Model file for the job. Use its own axes, mm. Face numbers are marked on the shaded views. A direction names the side the tool comes from. Coordinates: 2 decimals unless noted, no trailing zeros. Order: outer loops, then holes, each group sorted by start corner. A loop starts at its lowest first (then second) coordinate and runs counter-clockwise, first axis right, second up. Notation, with made-up numbers: M 84,5.25 L 128,5.25 A30 cw 128,38.25 Z; hole C 63,-14.75 d8. An arc over 180 degrees is marked long. Return JSON: item names as keys, results as strings.
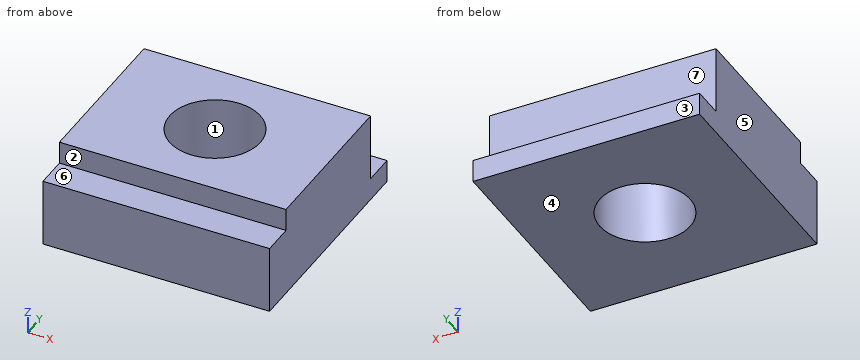
```python
from build123d import *

# Parameters (mm, degrees)
F0_W     = 50
F0_H     = 20
F1_DEPTH = 50
F2_W     = 7
F2_H     = 5
F2_H_2   = 15
F3_DEPTH = 50
F4_R     = 10
F5_DEPTH = 20


with BuildPart() as f1:
    # F0 (on Right) → F1 (new body)
    with BuildSketch(Plane.YZ):
        with Locations((25, 10)):
            Rectangle(F0_W, F0_H)
    extrude(amount=F1_DEPTH)

    # F2 (on face) → F3 (cut)
    with BuildSketch(Plane.YZ.offset(50)):
        with Locations((3.5, 17.5)):
            Rectangle(F2_W, F2_H)
        with Locations((46.5, 12.5)):
            Rectangle(F2_W, F2_H_2)
    extrude(amount=-F3_DEPTH, mode=Mode.SUBTRACT)

    # F4 (on face) → F5 (cut)
    with BuildSketch(Plane.XY.offset(20)):
        with Locations((25, 25)):
            Circle(F4_R)
    extrude(amount=-F5_DEPTH, mode=Mode.SUBTRACT)


solid = f1.part
```
Item 1: Drop flat-ended pins along their axis: pin 1 Ø16 at (x, y) = (25, 25) entering from +Z; pin 2 Ø2 at (x, z) = (27, 18) entering from -Y; pin 3 Ø5.5 at (x, y) = (34, 47.5) entering from +Z; pin 4 Ø2 at (x, y) = (34.5, 3) entering from +Z. Give the stop position or say it passes through.
Check result:
{"pin 1": "passes through", "pin 2": "stops at y = 7", "pin 3": "stops at z = 5", "pin 4": "stops at z = 15"}
Item 2: Saw through at A-A (y = 25). Write the cut outline in (x, z), and give its area (3 significant figures).
Check result:
{"outline": "M 0,0 L 15,0 L 15,20 L 0,20 Z; M 35,0 L 50,0 L 50,20 L 35,20 Z", "area": "600 mm2"}
Item 3: 3-axis set-ups, long thin cutter, end or side, ignore diameter. For the marked faces 5, 6 and 7: which of +Z, -Z, +X, -X, +Y, -Y reach the whole face in a straight line?
Check result:
{"face 5": "+Z, -Z, -X, +Y, -Y", "face 6": "+Z, +X, -X, -Y", "face 7": "+Z, +X, -X, +Y"}
Item 4: Saw through at B-B (x = 25). Write the cut outline in (y, z), and give its area (3 significant figures).
Check result:
{"outline": "M 0,0 L 15,0 L 15,20 L 7,20 L 7,15 L 0,15 Z; M 35,0 L 50,0 L 50,5 L 43,5 L 43,20 L 35,20 Z", "area": "460 mm2"}
Item 5: Saw through at D-D (x = 11.5). Write the cut outline in (y, z).
Check result:
{"outline": "M 0,0 L 50,0 L 50,5 L 43,5 L 43,20 L 7,20 L 7,15 L 0,15 Z"}
Item 6: Wall check: line 1 (Y direction, x = 25, z = 8.75); line 2 (Y direction, x = 38, z = 14.75); line 3 (Y direction, x = 25, z = 15.25). Give the ranges that are in metal, low to high.
Check result:
{"line 1": "y = 0 to 15, 35 to 43", "line 2": "y = 0 to 43", "line 3": "y = 7 to 15, 35 to 43"}
Item 7: Saw through at C-C (z = 7). Write the cut outline in (x, y).
Check result:
{"outline": "M 0,0 L 50,0 L 50,43 L 0,43 Z; hole C 25,25 d20"}
Item 8: Pull direction Y, two halves, no side cores. Call the marked faces 1, 2, 3 and 4: +Y half, -Y half, draft (parallel to the pull), parting line (faces both ways), or undercut.
Check result:
{"face 1": "undercut", "face 2": "-Y half", "face 3": "+Y half", "face 4": "draft"}
